Here's the drawing with two shaded views (mm, measured from the low corner). I have some questions. Give positions to 0.01 mm unless a question says otherwise; leave off trailing zeros. Order: outer loops, then holes, each group sorted by start corner. A loop starts at its lowest first (then second) coordinate and runs counter-clockwise, first axis right, second up. Notation, with made-up numbers: M 0.25,76.5 L 11.25,76.5 A26 cw 11.25,101.5 Z; hole C 78.5,46 d1. An arc over 180 degrees is marked long. Write each question's results on one line, items separated by ' | '.
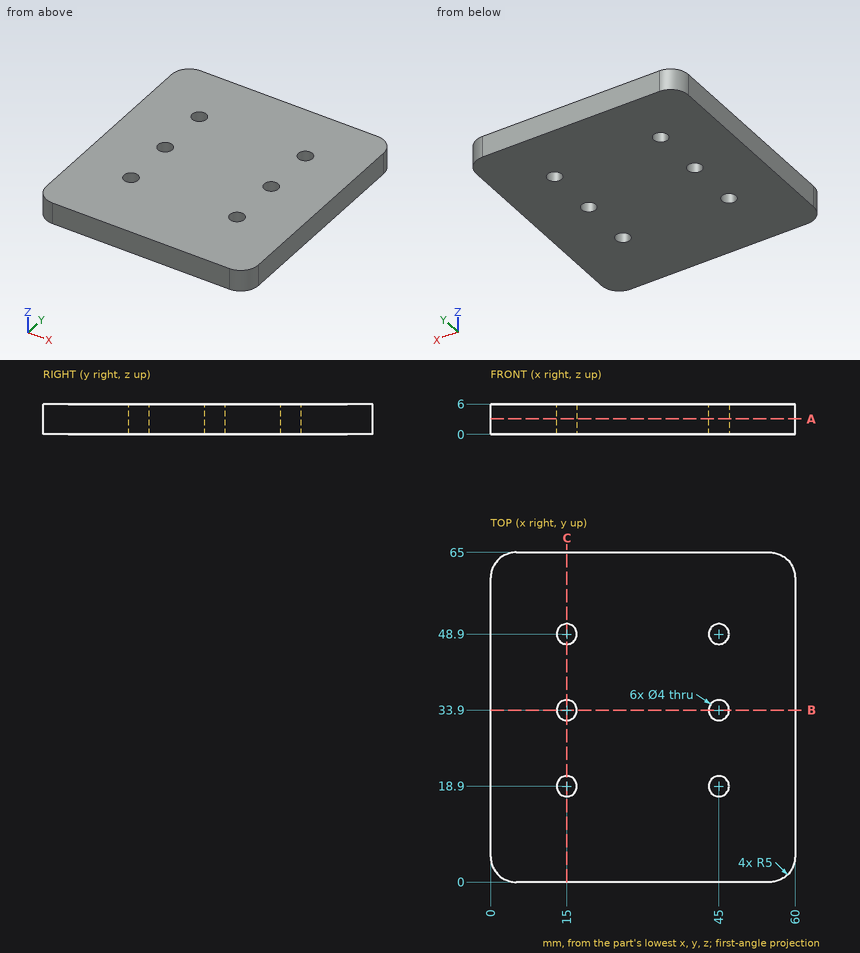
(1) I need wall thicknesses on L1, parallel to Y at x = 45, z = 2.55; L2, parallel to X at y = 50, z = 1.5; L3, parallel to Y at x = 16.5, z = 0.6. Which ranges of each line are inside material? Lowest first, please. Write a range as from..to.
Data:
L1: y = 0..16.9, 20.9..31.9, 35.9..46.9, 50.9..65 | L2: x = 0..13.33, 16.67..43.33, 46.67..60 | L3: y = 0..17.58, 20.22..32.58, 35.22..47.58, 50.22..65
(2) Imagine slicing it at B-B, the plane y = 33.9. Write out the boundary of the cut face in (x, z), plus the area to 3 significant figures.
Data:
outline: M 0,0 L 13,0 L 13,6 L 0,6 Z; M 17,0 L 43,0 L 43,6 L 17,6 Z; M 47,0 L 60,0 L 60,6 L 47,6 Z | area: 312 mm2
(3) Imagine slicing it at C-C, the plane x = 15. Write out the boundary of the cut face in (y, z), plus the area to 3 significant figures.
Data:
outline: M 0,0 L 16.9,0 L 16.9,6 L 0,6 Z; M 20.9,0 L 31.9,0 L 31.9,6 L 20.9,6 Z; M 35.9,0 L 46.9,0 L 46.9,6 L 35.9,6 Z; M 50.9,0 L 65,0 L 65,6 L 50.9,6 Z | area: 318 mm2
(4) Imagine slicing it at A-A, the plane z = 3.05. Write out the boundary of the cut face in (x, y), plus the area to 3 significant figures.
Data:
outline: M 0,5 A5 ccw 5,0 L 55,0 A5 ccw 60,5 L 60,60 A5 ccw 55,65 L 5,65 A5 ccw 0,60 Z; hole C 15,18.9 d4; hole C 15,33.9 d4; hole C 15,48.9 d4; hole C 45,18.9 d4; hole C 45,33.9 d4; hole C 45,48.9 d4 | area: 3,800 mm2
